Autodesk Inventor part; units mm, degrees
ref_plane "YZ Plane" through (0, 0, 0) normal (1, 0, 0) x (0, 1, 0)
ref_plane "XZ Plane" through (0, 0, 0) normal (0, 1, 0) x (-1, 0, 0)
ref_plane "XY Plane" through (0, 0, 0) normal (0, 0, 1) x (1, 0, 0)
sketch "Esquisse1" plane through (0, 0, 0) normal (0, 1, 0) x (-1, 0, 0)
  circle A0 centre (0, 0) radius 22
  dimension "d0" = 44
extrude "Extrusion1" add sketch "Esquisse1" along normal blind 2.4
sketch "Esquisse2" plane through (0, 2.4, 0) normal (0, 1, 0) x (1, 0, 0)
  circle A0 centre (0, 0) radius 22
  circle A1 centre (0, 0) radius 11
  dimension "d3" = 22
extrude "Extrusion2" add sketch "Esquisse2" along normal blind 19 contours A1
sketch "Esquisse4" plane through (0, 0, 0) normal (0, -1, 0) x (1, 0, 0)
  circle A0 centre (0, 0) radius 22
  circle A1 centre (0, 17.5) radius 2.75
  dimension "d6" = 5.5
  dimension "d7" = 17.5
extrude "Extrusion3" cut sketch "Esquisse4" against normal through all contours A1
pattern_circular "Réseau circulaire1" count 3 over 360 about axis through (0, 2.4, 0) along (0, 1, 0) of "Extrusion3"
sketch "Esquisse5" plane through (0, 0, 0) normal (0, -1, 0) x (1, 0, 0)
  circle A0 centre (0, 0) radius 22
  circle A1 centre (0, 0) radius 3.9
  dimension "d13" = 7.8
extrude "Extrusion4" add sketch "Esquisse5" along normal blind 9 contours A1
properties part number "SRC022" material "Plastique ABS"
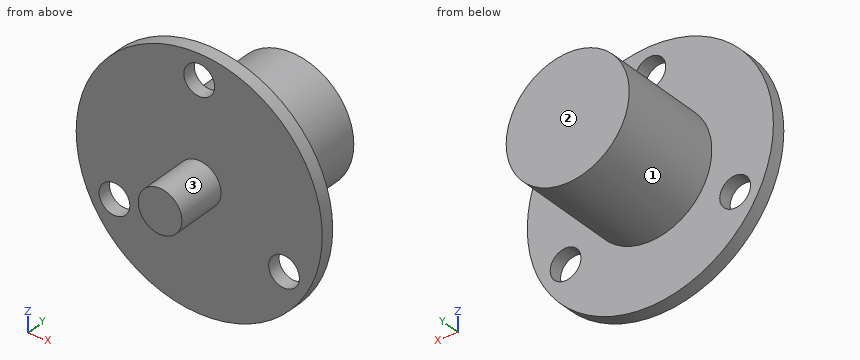
Check sheet for the modelled part. Datum: model origin and axes. Units: mm. Face numbers are marked on the shaded views. A direction names the side the tool comes from. Give positions to 0.01 mm unless a question says otherwise; leave off trailing zeros. Loops run counter-clockwise (first coordinate to the right, second up) from the corner with the lowest first, then second, coordinate; pieces in that order, holes last. Notation, with made-up numbers: M 70.25,70 L 128.25,70 A20 cw 128.25,84 Z; hole C -26.5,33 d4. An arc over 180 degrees is marked long. Use a Markdown table: item, result. Add a question column.
Q1. Scan lines: line 1 along X through (y, z) = (1, -8); line 2 along Y through (x, z) = (8, 14); line 3 along Z through (x, y) = (0, 1.2). Record each from-to range of solid material in increasing order. Write a range as [from, to].
Q2. Sectioned sample at A-A, the plane x = 0. Record the cut outline in (y, z), then the cut area to 3 significant figures.
Q3. Sectioned sample at B-B, the plane z = 0. Record the cut outline in (x, y), then the cut area to 3 significant figures.
Q4. Sectioned sample at C-C, the plane z = 17.5. Record the cut outline in (x, y), then the cut area to 3 significant figures.
Q5. Go/stop test with flat-tipped pins: pin 1 (2 mm diameter, centred on y = 1.5, z = -10.5, fed in from +X); pin 2 (7 mm diameter, centred on x = 0, z = 17.5, fed in from +Y); pin 3 (7 mm diameter, centred on x = -15.16, z = -8.75, fed in from -Y); pin 4 (1 mm diameter, centred on x = -14, y = 3, fed in from -Z). Record where each tip stops, or that it passes through.
Q6. Sectioned sample at D-D, the plane x = -13.5. Record the cut outline in (y, z), then the cut area to 3 significant figures.
Q7. Tool access check on the marked faces 1, 2 and 3. Record the directions out of +Z, -Z, +X, -X, +Y, -Y that give a thin tool (end or side, any length) a straight path to the whole face; none if there is none.
Verdict:
| question | item | result |
|---|---|---|
| 1 | line 1 | [-20.49, -17.8], [-12.51, 12.51], [17.8, 20.49] |
| 1 | line 2 | [0, 2.4] |
| 1 | line 3 | [-22, 14.75], [20.25, 22] |
| 2 | outline | M -9,-3.9 L 0,-3.9 L 0,-22 L 2.4,-22 L 2.4,-11 L 21.4,-11 L 21.4,11 L 2.4,11 L 2.4,14.75 L 0,14.75 L 0,3.9 L -9,3.9 Z; M 0,20.25 L 2.4,20.25 L 2.4,22 L 0,22 Z |
| 2 | area | 581 mm^2 |
| 3 | outline | M -22,0 L -3.9,0 L -3.9,-9 L 3.9,-9 L 3.9,0 L 22,0 L 22,2.4 L 11,2.4 L 11,21.4 L -11,21.4 L -11,2.4 L -22,2.4 Z |
| 3 | area | 594 mm^2 |
| 4 | outline | M -13.33,0 L -2.75,0 L -2.75,2.4 L -13.33,2.4 Z; M 2.75,0 L 13.33,0 L 13.33,2.4 L 2.75,2.4 Z |
| 4 | area | 50.8 mm^2 |
| 5 | pin 1 | x = 19.84 |
| 5 | pin 2 | y = 2.4 |
| 5 | pin 3 | y = 0 |
| 5 | pin 4 | through |
| 6 | outline | M 0,-17.37 L 2.4,-17.37 L 2.4,-10.95 L 0,-10.95 Z; M 0,-6.55 L 2.4,-6.55 L 2.4,17.37 L 0,17.37 Z |
| 6 | area | 72.8 mm^2 |
| 7 | face 1 | +Y |
| 7 | face 2 | +Z, -Z, +X, -X, +Y |
| 7 | face 3 | -Y |
